Build history of the part. All positions in model axes, mm. A direction names the side the tool comes from. Round coordinates to 2 decimals unless told otherwise and drop trailing zeros. Write each loop counter-clockwise with the first axis right and the second up, starting at its lowest first coordinate (ties: lowest second). Pieces come first, ordered by that corner, then holes. Notation, with made-up numbers: M 25,12 L 66,12 A24 ccw 66,39 Z; hole C 24.5,-36 d10. An arc over 180 degrees is marked long. Use a Markdown table: item, result.
from build123d import *

# Parameters (mm, degrees)
BOSS_EXTRUDE1_DEPTH            = 100
CUT_EXTRUDE3_DEPTH             = 202.556443707
CUT_EXTRUDE3_DEPTH_BACK        = 202.556443707
SKETCH4_4_R                    = 9.85
CUT_EXTRUDE4_DEPTH             = 3
CUT_EXTRUDE5_START             = 103
SKETCH4_6_R                    = 9.85
CUT_EXTRUDE5_DEPTH             = 103
CUT_EXTRUDE6_REACH             = 206.206
SKETCH5_R                      = 2.25
CUT_EXTRUDE6_DIRECTION_2_DEPTH = 205.205778567
CUT_EXTRUDE7_REACH             = 201.841
SKETCH6_R                      = 2.25
SKETCH7_W                      = 12
SKETCH7_H                      = 15
CUT_EXTRUDE8_DEPTH             = 197.242821038
FILLET3_R                      = 2.5
FILLET4_R                      = 2.5
FILLET6_R                      = 5
CUT_EXTRUDE9_DEPTH             = 197.242821038
CUT_EXTRUDE9_DEPTH_BACK        = 197.242821038
SKETCH8_W                      = 5
SKETCH8_H                      = 100
CUT_EXTRUDE10_REACH            = 136.228
SKETCH11_R                     = 1.75


with BuildPart() as part:
    # Sketch1 → Boss-Extrude1 (new body)
    with BuildSketch(Plane.XY):
        Polygon((-10.600610125, 140), (-15.600610125, 140), (-15.600610125, -5), (94.399389875, -5), (94.399389875, 140), (89.399389875, 140), (89.399389875, 0), (-10.600610125, 0), align=None)
    extrude(amount=-BOSS_EXTRUDE1_DEPTH)

    # Sketch4 → Cut-Extrude3 (cut, two sides: drawn at the far end of the back side and taken through both)
    with BuildSketch(Plane.ZY.offset(-89.399389875).offset(-CUT_EXTRUDE3_DEPTH_BACK)):
        with BuildLine():
            ThreePointArc((-89.05, 45), (-82.05, 38), (-75.05, 45))
            Line((-75.05, 45), (-82.05, 45))
            Line((-82.05, 45), (-89.05, 45))
        make_face()
        with BuildLine():
            Line((-82.05, 45), (-75.05, 45))
            ThreePointArc((-75.05, 45), (-82.05, 52), (-89.05, 45))
            Line((-89.05, 45), (-82.05, 45))
        make_face()
        with BuildLine():
            ThreePointArc((-57, 45), (-50, 38), (-43, 45))
            Line((-43, 45), (-50, 45))
            Line((-50, 45), (-57, 45))
        make_face()
        with BuildLine():
            Line((-50, 45), (-43, 45))
            ThreePointArc((-43, 45), (-50, 52), (-57, 45))
            Line((-57, 45), (-50, 45))
        make_face()
        with BuildLine():
            ThreePointArc((-24.95, 45), (-17.95, 38), (-10.95, 45))
            Line((-10.95, 45), (-17.95, 45))
            Line((-17.95, 45), (-24.95, 45))
        make_face()
        with BuildLine():
            Line((-17.95, 45), (-10.95, 45))
            ThreePointArc((-10.95, 45), (-17.95, 52), (-24.95, 45))
            Line((-24.95, 45), (-17.95, 45))
        make_face()
    extrude(amount=CUT_EXTRUDE3_DEPTH + CUT_EXTRUDE3_DEPTH_BACK, mode=Mode.SUBTRACT)

    # Sketch4<4> → Cut-Extrude4 (cut)
    with BuildSketch(Plane.ZY.offset(-89.399389875)):
        with Locations((-50, 45)):
            Circle(SKETCH4_4_R)
        with Locations((-82.05, 45)):
            Circle(SKETCH4_4_R)
        with Locations((-17.95, 45)):
            Circle(SKETCH4_4_R)
    extrude(amount=-CUT_EXTRUDE4_DEPTH, mode=Mode.SUBTRACT)

    # Sketch4<6> → Cut-Extrude5 (cut)
    with BuildSketch(Plane.ZY.offset(-89.399389875).offset(CUT_EXTRUDE5_START)):
        with Locations((-50, 45)):
            Circle(SKETCH4_6_R)
        with Locations((-82.05, 45)):
            Circle(SKETCH4_6_R)
        with Locations((-17.95, 45)):
            Circle(SKETCH4_6_R)
    extrude(amount=-CUT_EXTRUDE5_DEPTH, mode=Mode.SUBTRACT)

    # Sketch5 → Cut-Extrude6 (cut, up to next)
    with BuildSketch(Plane.ZY.offset(15.600610125), mode=Mode.PRIVATE) as cut_extrude6_sk1:
        with Locations(Location((-78.75, 119.5, 0), (0, 0, 90))):
            Circle(SKETCH5_R)
    cut_extrude6_tool1 = extrude(cut_extrude6_sk1.sketch, amount=-CUT_EXTRUDE6_REACH, mode=Mode.PRIVATE) & part.part
    # Sketch5 → Cut-Extrude6 (cut, up to next)
    with BuildSketch(Plane.ZY.offset(15.600610125), mode=Mode.PRIVATE) as cut_extrude6_sk2:
        with Locations(Location((-21.25, 119.5, 0), (0, 0, 90))):
            Circle(SKETCH5_R)
    cut_extrude6_tool2 = extrude(cut_extrude6_sk2.sketch, amount=-CUT_EXTRUDE6_REACH, mode=Mode.PRIVATE) & part.part
    add(cut_extrude6_tool1.solids().sort_by_distance((-15.60061, 119.5, -78.75))[0], mode=Mode.SUBTRACT)
    add(cut_extrude6_tool2.solids().sort_by_distance((-15.60061, 119.5, -21.25))[0], mode=Mode.SUBTRACT)

    # Sketch5 → Cut-Extrude6 direction 2 (cut)
    with BuildSketch(Plane.ZY.offset(15.600610125)):
        with Locations(Location((-78.75, 119.5, 0), (0, 0, 90))):
            Circle(SKETCH5_R)
        with Locations(Location((-21.25, 119.5, 0), (0, 0, 90))):
            Circle(SKETCH5_R)
    extrude(amount=CUT_EXTRUDE6_DIRECTION_2_DEPTH, mode=Mode.SUBTRACT)

    # Sketch6 → Cut-Extrude7 (cut, up to next)
    with BuildSketch(Plane.XZ.offset(5), mode=Mode.PRIVATE) as cut_extrude7_sk1:
        with Locations(Location((71.899389875, -50, 0), (0, 0, 270))):
            Circle(SKETCH6_R)
    cut_extrude7_tool1 = extrude(cut_extrude7_sk1.sketch, amount=-CUT_EXTRUDE7_REACH, mode=Mode.PRIVATE) & part.part
    # Sketch6 → Cut-Extrude7 (cut, up to next)
    with BuildSketch(Plane.XZ.offset(5), mode=Mode.PRIVATE) as cut_extrude7_sk2:
        with Locations(Location((6.899389875, -50, 0), (0, 0, 270))):
            Circle(SKETCH6_R)
    cut_extrude7_tool2 = extrude(cut_extrude7_sk2.sketch, amount=-CUT_EXTRUDE7_REACH, mode=Mode.PRIVATE) & part.part
    add(cut_extrude7_tool1.solids().sort_by_distance((71.89939, -5, -50))[0], mode=Mode.SUBTRACT)
    add(cut_extrude7_tool2.solids().sort_by_distance((6.89939, -5, -50))[0], mode=Mode.SUBTRACT)

    # Sketch7 → Cut-Extrude8 (cut, through all)
    with BuildSketch(Plane(origin=(0, 0, 0), x_dir=(1, 0, 0), z_dir=(0, 1, 0))):
        Polygon((45.399389875, 100), (39.399389875, 100), (33.399389875, 100), (33.399389875, 85), (45.399389875, 85), align=None)
        with Locations((39.399389875, 7.5)):
            Rectangle(SKETCH7_W, SKETCH7_H)
    extrude(amount=-CUT_EXTRUDE8_DEPTH, mode=Mode.SUBTRACT)

    # Fillet3
    fillet3_edges = [part.edges().sort_by_distance(p)[0] for p in [
        (33.399389875, 0, -7.5),
        (33.399389875, -2.5, 0),
        (39.399389875, 0, -15),
        (33.399389875, -2.5, -15),
        (45.399389875, -5, -7.5),
        (45.399389875, -2.5, -15),
        (45.399389875, -2.5, 0),
        (33.399389875, -5, -7.5),
        (39.399389875, -5, -15),
        (45.399389875, 0, -7.5),
    ]]
    fillet(fillet3_edges, radius=FILLET3_R - 0.0001)  # a hair under: the kernel refuses the full size

    # Fillet4
    fillet4_edges = [part.edges().sort_by_distance(p)[0] for p in [
        (45.399389875, 0, -92.5),
        (45.399389875, -2.5, -100),
        (39.399389875, -5, -85),
        (45.399389875, -2.5, -85),
        (33.399389875, -5, -92.5),
        (33.399389875, -2.5, -85),
        (33.399389875, -2.5, -100),
        (45.399389875, -5, -92.5),
        (33.399389875, 0, -92.5),
        (39.399389875, 0, -85),
    ]]
    fillet(fillet4_edges, radius=FILLET4_R - 0.0001)  # a hair under: the kernel refuses the full size

    # Fillet6
    fillet6_edges = [part.edges().sort_by_distance(p)[0] for p in [
        (91.899389875, 140, -100),
        (-13.100610125, 140, -100),
        (-13.100610125, 140, 0),
        (91.899389875, 140, 0),
    ]]
    fillet(fillet6_edges, radius=FILLET6_R)

    # Sketch8 → Cut-Extrude9 (cut, two sides: drawn at the far end of the back side and taken through both)
    with BuildSketch(Plane(origin=(0, 0, 0), x_dir=(1, 0, 0), z_dir=(0, 1, 0)).offset(-CUT_EXTRUDE9_DEPTH_BACK)):
        with Locations((-13.100610125, 50)):
            Rectangle(SKETCH8_W, SKETCH8_H)
        with Locations((91.899389875, 50)):
            Rectangle(SKETCH8_W, SKETCH8_H)
    extrude(amount=CUT_EXTRUDE9_DEPTH + CUT_EXTRUDE9_DEPTH_BACK, mode=Mode.SUBTRACT)

    # Sketch11 → Cut-Extrude10 (cut, up to next)
    with BuildSketch(Plane(origin=(0, 0, 0), x_dir=(1, 0, 0), z_dir=(0, 1, 0)), mode=Mode.PRIVATE) as cut_extrude10_sk1:
        with Locations(Location((80.899389875, 65, 0), (0, 0, 270))):
            Circle(SKETCH11_R)
    cut_extrude10_tool1 = extrude(cut_extrude10_sk1.sketch, amount=-CUT_EXTRUDE10_REACH, mode=Mode.PRIVATE) & part.part
    # Sketch11 → Cut-Extrude10 (cut, up to next)
    with BuildSketch(Plane(origin=(0, 0, 0), x_dir=(1, 0, 0), z_dir=(0, 1, 0)), mode=Mode.PRIVATE) as cut_extrude10_sk2:
        with Locations(Location((80.899389875, 35, 0), (0, 0, 270))):
            Circle(SKETCH11_R)
    cut_extrude10_tool2 = extrude(cut_extrude10_sk2.sketch, amount=-CUT_EXTRUDE10_REACH, mode=Mode.PRIVATE) & part.part
    # Sketch11 → Cut-Extrude10 (cut, up to next)
    with BuildSketch(Plane(origin=(0, 0, 0), x_dir=(1, 0, 0), z_dir=(0, 1, 0)), mode=Mode.PRIVATE) as cut_extrude10_sk3:
        with Locations(Location((-2.100610125, 35, 0), (0, 0, 270))):
            Circle(SKETCH11_R)
    cut_extrude10_tool3 = extrude(cut_extrude10_sk3.sketch, amount=-CUT_EXTRUDE10_REACH, mode=Mode.PRIVATE) & part.part
    # Sketch11 → Cut-Extrude10 (cut, up to next)
    with BuildSketch(Plane(origin=(0, 0, 0), x_dir=(1, 0, 0), z_dir=(0, 1, 0)), mode=Mode.PRIVATE) as cut_extrude10_sk4:
        with Locations(Location((-2.100610125, 65, 0), (0, 0, 270))):
            Circle(SKETCH11_R)
    cut_extrude10_tool4 = extrude(cut_extrude10_sk4.sketch, amount=-CUT_EXTRUDE10_REACH, mode=Mode.PRIVATE) & part.part
    add(cut_extrude10_tool1.solids().sort_by_distance((80.89939, 0, -65))[0], mode=Mode.SUBTRACT)
    add(cut_extrude10_tool2.solids().sort_by_distance((80.89939, 0, -35))[0], mode=Mode.SUBTRACT)
    add(cut_extrude10_tool3.solids().sort_by_distance((-2.10061, 0, -35))[0], mode=Mode.SUBTRACT)
    add(cut_extrude10_tool4.solids().sort_by_distance((-2.10061, 0, -65))[0], mode=Mode.SUBTRACT)


solid = part.part
Q1. Which spindle directions (+Z, -Z, +X, -X, +Y, -Y) get a long thin tool onto all of the face, cutting with end or side? Do faces 1 (the cylindrical face through (32.648, -0.713, -6.338)), 2 (the cylindrical face through (32.4, -2.5, -99.5)), 3 (the cylindrical face through (46.151, -0.713, -93.837)), 4 (the cylindrical face through (46.151, -4.287, -6.163)). Say none if no direction does.
Response values:
| item | result |
|---|---|
| face 1 | +Z, +Y |
| face 2 | -Z, +Y, -Y |
| face 3 | -Z, +Y |
| face 4 | +Z, -Y |
Q2. Cut at C-C on z = -50. Give the cut face in (x, y), and give its area (3 significant figures).
Response values:
| item | result |
|---|---|
| outline | M -10.6,-5 L 4.65,-5 L 4.65,0 L -10.6,0 Z; M 9.15,-5 L 69.65,-5 L 69.65,0 L 9.15,0 Z; M 74.15,-5 L 89.4,-5 L 89.4,0 L 74.15,0 Z |
| area | 455 mm2 |
Q3. Cut at B-B on z = -35. Give the cut face in (x, y), and give its area (3 significant figures).
Response values:
| item | result |
|---|---|
| outline | M -10.6,-5 L -3.85,-5 L -3.85,0 L -10.6,0 Z; M -0.35,-5 L 79.15,-5 L 79.15,0 L -0.35,0 Z; M 82.65,-5 L 89.4,-5 L 89.4,0 L 82.65,0 Z |
| area | 465 mm2 |
Q4. Drill centre lines: L1, parallel to X at y = -2.2, z = -35; L2, parallel to X at y = -1.5, z = -49.5; L3, parallel to Z at x = 81.5, y = -2.7. Where is each one in solid material? Low to high.
Response values:
| item | result |
|---|---|
| L1 | x = -10.6 to -3.85, -0.35 to 79.15, 82.65 to 89.4 |
| L2 | x = -10.6 to 4.71, 9.09 to 69.71, 74.09 to 89.4 |
| L3 | z = -100 to -66.64, -63.36 to -36.64, -33.36 to 0 |
Q5. Drop flat-ended pins along their axis: P1, Ø3, axis at x = -2.1, z = -35, coming from the +Y side; P2, Ø10, axis at x = 15, z = -88.5, coming from the +Y side. Give the stop position or say it passes through.
Response values:
| item | result |
|---|---|
| P1 | passes through |
| P2 | stops at y = 0 |
Q6. Two-plate mould, pull along Z, no slides. Class faces 5 (the cylindrical face through (6.998, -2.535, -47.752)), 6 (the cylindrical face through (46.488, -2.535, -99.564)), 7 (the flat face through (10, -2, 0)): +Z half, -Z half, draft (parallel to the pull), parting line (faces both ways), or undercut.
Response values:
| item | result |
|---|---|
| face 5 | undercut |
| face 6 | -Z half |
| face 7 | +Z half |
